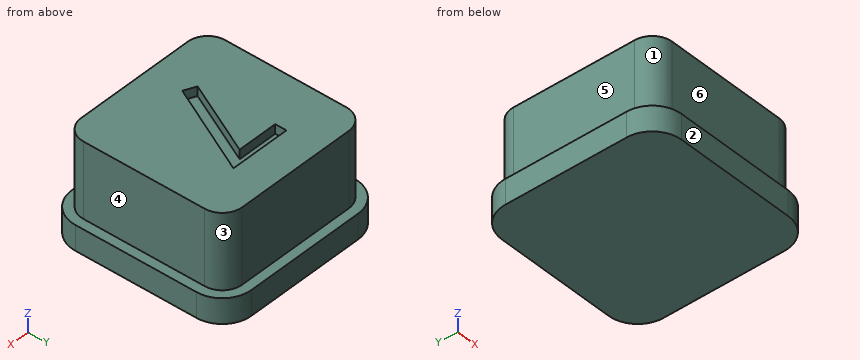
```python
from build123d import *

# Parameters (mm, degrees)
F1_DEPTH = 2
F2_DEPTH = 8
F3_DEPTH = 7.25


with BuildPart() as f1:
    # F0 (on Top) → F1 (new body)
    with BuildSketch(Plane.XY):
        with BuildLine():
            Line((4.85, 7.2), (-4.85, 7.2))
            ThreePointArc((-4.85, 7.2), (-6.511701, 6.511701), (-7.2, 4.85))
            Line((-7.2, 4.85), (-7.2, -4.85))
            ThreePointArc((-7.2, -4.85), (-6.511701, -6.511701), (-4.85, -7.2))
            Line((-4.85, -7.2), (4.85, -7.2))
            ThreePointArc((4.85, -7.2), (6.511701, -6.511701), (7.2, -4.85))
            Line((7.2, -4.85), (7.2, 4.85))
            ThreePointArc((7.2, 4.85), (6.511701, 6.511701), (4.85, 7.2))
        make_face()
        with BuildLine():
            ThreePointArc((6.45, -4.85), (5.981371, -5.981371), (4.85, -6.45))
            Line((4.85, -6.45), (-4.85, -6.45))
            ThreePointArc((-4.85, -6.45), (-5.981371, -5.981371), (-6.45, -4.85))
            Line((-6.45, -4.85), (-6.45, 4.85))
            ThreePointArc((-6.45, 4.85), (-5.981371, 5.981371), (-4.85, 6.45))
            Line((-4.85, 6.45), (4.85, 6.45))
            ThreePointArc((4.85, 6.45), (5.981371, 5.981371), (6.45, 4.85))
            Line((6.45, 4.85), (6.45, -4.85))
        make_face(mode=Mode.SUBTRACT)
    extrude(amount=F1_DEPTH)

    # F0 (on Top) → F2 (join)
    with BuildSketch(Plane.XY):
        with BuildLine():
            Line((-4.85, -6.45), (4.85, -6.45))
            ThreePointArc((4.85, -6.45), (5.981371, -5.981371), (6.45, -4.85))
            Line((6.45, -4.85), (6.45, 4.85))
            ThreePointArc((6.45, 4.85), (5.981371, 5.981371), (4.85, 6.45))
            Line((4.85, 6.45), (-4.85, 6.45))
            ThreePointArc((-4.85, 6.45), (-5.981371, 5.981371), (-6.45, 4.85))
            Line((-6.45, 4.85), (-6.45, -4.85))
            ThreePointArc((-6.45, -4.85), (-5.981371, -5.981371), (-4.85, -6.45))
        make_face()
        Polygon((-1.11168, -3.598019), (-2.034495, -3.186817), (0.824795, 2.699112), (-2.412227, 2.699112), (-2.412227, 3.598019), (2.412227, 3.598019), align=None, mode=Mode.SUBTRACT)
    extrude(amount=F2_DEPTH)

    # F0 (on Top) → F3 (join)
    with BuildSketch(Plane.XY):
        Polygon((0.824795, 2.699112), (-2.034495, -3.186817), (-1.11168, -3.598019), (2.412227, 3.598019), (-2.412227, 3.598019), (-2.412227, 2.699112), align=None)
    extrude(amount=F3_DEPTH)


solid = f1.part
```
Part model, mm, in its own coordinate system. Face numbers are marked on the shaded views. A direction names the side the tool comes from. Round coordinates to 2 decimals unless told otherwise and drop trailing zeros. Loops run counter-clockwise (first coordinate to the right, second up) from the corner with the lowest first, then second, coordinate; pieces in that order, holes last.
Item 1: Cut at A-A, the plane x = 4. Give the cut face in (y, z).
Item 2: Mould opens along X. For the marked faces 1, 2 and 3 say: +X half, -X half, draft (parallel to the pull), parting line (faces both ways), or undercut.
Item 3: 3-axis set-ups, long thin cutter, end or side, ignore diameter. For the marked faces 4, 5 and 6: which of +Z, -Z, +X, -X, +Y, -Y reach the whole face in a straight line?
Item 4: Drill centre lines: line 1 (Y direction, x = 3.25, z = 6.75); line 2 (X direction, y = 2.25, z = 7.5). Where is each one in solid material? Low to high.
Item 5: Cut at D-D, the plane y = -2.75. Give the cut face in (x, z), then the cut area to 3 significant figures.
Item 6: Cut at B-B, the plane y = -0.25. Give the cut face in (x, z).
Item 7: Drop flat-ended pins along their axis: P1, Ø1.8, axis at x = 0, z = 5, coming from the -Y side; P2, Ø1.8, axis at x = 1, z = 4.5, coming from the +Y side; P3, Ø2, axis at y = -3, z = 7, coming from the +X side. Give the stop position or say it passes through.
Item 8: Cut at C-C, the plane z = 4.75. Give the cut face in (x, y).
A:
1. outline: (-7.2, 0) - (7.2, 0) - (7.2, 2) - (6.45, 2) - (6.45, 8) - (-6.45, 8) - (-6.45, 2) - (-7.2, 2) - close
2. face 1: -X half
2. face 2: draft
2. face 3: +X half
3. face 4: +Z, +X, +Y, -Y
3. face 5: +Z, -X, +Y, -Y
3. face 6: +Z, +X, -X, -Y
4. line 1: y = -6.45 to 6.45
4. line 2: x = -6.45 to 0.61, 1.75 to 6.45
5. outline: (-7.2, 0) - (7.2, 0) - (7.2, 2) - (6.45, 2) - (6.45, 8) - (-0.7, 8) - (-0.7, 7.25) - (-1.82, 7.25) - (-1.82, 8) - (-6.45, 8) - (-6.45, 2) - (-7.2, 2) - close
5. area: 105 mm2
6. outline: (-7.2, 0) - (7.2, 0) - (7.2, 2) - (6.45, 2) - (6.45, 8) - (0.53, 8) - (0.53, 7.25) - (-0.61, 7.25) - (-0.61, 8) - (-6.45, 8) - (-6.45, 2) - (-7.2, 2) - close
7. P1: stops at y = -6.45
7. P2: stops at y = 6.45
7. P3: stops at x = 6.45
8. outline: (-6.45, -4.85) arc R1.6 ccw to (-4.85, -6.45) - (4.85, -6.45) arc R1.6 ccw to (6.45, -4.85) - (6.45, 4.85) arc R1.6 ccw to (4.85, 6.45) - (-4.85, 6.45) arc R1.6 ccw to (-6.45, 4.85) - close
